from build123d import *

# Parameters (mm, degrees)
BOSS_EXTRUDE1_DEPTH     = 50
CUT_EXTRUDE1_DEPTH      = 80
SKETCH4_W               = 30
SKETCH4_H               = 117.064102809
CUT_EXTRUDE2_DEPTH      = 11.624305452
CUT_EXTRUDE2_DEPTH_BACK = 260


with BuildPart() as part:
    # Sketch1 → Boss-Extrude1 (new body)
    with BuildSketch(Plane.XY):
        with BuildLine():
            Line((-40.25, 0), (-47.5, 0))
            Line((-47.5, 0), (-47.5, -6.5))
            Line((-47.5, -6.5), (-50.5, -6.5))
            Line((-50.5, -6.5), (-142.624305452, -290))
            Line((-142.624305452, -290), (142.624305452, -290))
            Line((142.624305452, -290), (50.5, -6.5))
            Line((50.5, -6.5), (47.5, -6.5))
            Line((47.5, -6.5), (47.5, 0))
            Line((47.5, 0), (40.25, 0))
            ThreePointArc((40.25, 0), (0, -40.25), (-40.25, 0))
        make_face()
    extrude(amount=BOSS_EXTRUDE1_DEPTH)

    # Sketch2 → Cut-Extrude1 (cut)
    with BuildSketch(Plane.XY.offset(50)):
        Polygon((-123.602681001, -280), (-98.393052146, -202.420801488), (-53.602681001, -280), align=None)
        Polygon((48.863385573, -50), (93.402839801, -187.064102809), (39.746274541, -280), (-39.746274541, -280), (-93.402839801, -187.064102809), (-48.863385573, -50), align=None)
        Polygon((123.602681001, -280), (53.602681001, -280), (98.393052146, -202.420801488), align=None)
    extrude(amount=-CUT_EXTRUDE1_DEPTH, mode=Mode.SUBTRACT)

    # Sketch4 → Cut-Extrude2 (cut, two sides)
    with BuildSketch(Plane(origin=(132, 0, 0), x_dir=(0, 0, -1), z_dir=(1, 0, 0))) as cut_extrude2_sk:
        with Locations((-25, -118.532051405)):
            Rectangle(SKETCH4_W, SKETCH4_H)
    extrude(amount=CUT_EXTRUDE2_DEPTH, mode=Mode.SUBTRACT)
    extrude(cut_extrude2_sk.sketch, amount=-CUT_EXTRUDE2_DEPTH_BACK, mode=Mode.SUBTRACT)


solid = part.part
CAD build for the part. Positions are in the model's coordinates, mm. A direction names the side the tool comes from. Round coordinates to 2 decimals unless told otherwise and drop trailing zeros. Order: outer loops, then holes, each group sorted by start corner. A loop starts at its lowest first (then second) coordinate and runs counter-clockwise, first axis right, second up. Notation, with made-up numbers: M 66.5,69 L 109.5,69 A14 cw 109.5,76 Z; hole C 57,-10.5 d6. An arc over 180 degrees is marked long. Use one line per item in the form item = value.
Q1. Saw through at A-A on z = 29.5. State how many separate pieces and enclosed holes the cut face has, then the cut area to 3 significant figures.
Recorded:
separate_pieces = 2
enclosed_holes = 2
area = 11,800 mm^2
Q2. Probe L1, parallel to X at y = -269.5, z = 42.5; L2, parallel to Y at x = 14, z = 9; L3, parallel to X at y = -232, z = 29. List the from-to ranges inside material, lowest first.
Recorded:
L1 = -135.96 to -120.19, -59.66 to -45.81, 45.81 to 59.66, 120.19 to 135.96
L2 = -290 to -280, -50 to -37.74
L3 = -123.78 to -108, -81.32 to -67.46, 67.46 to 81.32, 108 to 123.78
Q3. Saw through at C-C on y = -194.5. Give the cut face in (x, z).
Recorded:
outline = M -111.59,0 L -89.11,0 L -89.11,50 L -111.59,50 Z; M 89.11,0 L 111.59,0 L 111.59,50 L 89.11,50 Z
Q4. Saw through at B-B on x = 0. Give the cut face in (y, z).
Recorded:
outline = M -290,0 L -280,0 L -280,50 L -290,50 Z; M -50,0 L -40.25,0 L -40.25,50 L -50,50 Z
Q5. Flat gauge pins, fed straight in: P1, Ø16, axis at x = 91, y = -126, coming from the +Z side; P2, Ø7, axis at y = -3.5, z = 31, coming from the -X side; P3, Ø6, axis at y = -192.5, z = 45, coming from the -X side; P4, Ø1.5, axis at x = -48.5, z = 21.5, coming from the +Y side. Where does each tip first touch, or does it go through?
Recorded:
P1 = 50
P2 = -50.66
P3 = -111.92
P4 = -6.5
Q6. Which spindle directions (+Z, -Z, +X, -X, +Y, -Y) get a long thin tool onto all of the face, cutting with end or side? Do faces 3 (the flat face through (-81, -119, 40)), 4 (the flat face through (-44, 0, 25)), 5 (the flat face through (98, -177.064, 25)), 6 (the flat face through (75.684, -241.753, 25.35)), 7 (the flat face through (-47.5, -3, 25)). Say none if no direction does.
Recorded:
face_3 = +X, -X
face_4 = +Z, -Z, +X, -X, +Y
face_5 = +X, -X, +Y
face_6 = +Z, -Z
face_7 = +Z, -Z, -X, +Y
Q7. Two-plate mould, pull along Z, no slides. Class faces 1 (the flat face through (60, -60, 25)), 2 (the flat face through (-76.31, -240.67, 25.35)): +Z half, -Z half, draft (parallel to the pull), parting line (faces both ways), or undercut.
Recorded:
face_1 = undercut
face_2 = draft
Q8. Saw through at D-D on y = -260. Give the cut face in (x, z), then the cut area to 3 significant figures.
Recorded:
outline = M -132.88,0 L -117.1,0 L -117.1,50 L -132.88,50 Z; M -65.15,0 L -51.29,0 L -51.29,50 L -65.15,50 Z; M 51.29,0 L 65.15,0 L 65.15,50 L 51.29,50 Z; M 117.1,0 L 132.88,0 L 132.88,50 L 117.1,50 Z
area = 2,960 mm^2
